Check sheet for the modelled part. Datum: model origin and axes. Units: mm. A direction names the side the tool comes from. Coordinates: 2 decimals unless noted, no trailing zeros. Loops run counter-clockwise (first coordinate to the right, second up) from the corner with the lowest first, then second, coordinate; pieces in that order, holes last. Notation, with made-up numbers: (-6.75, 60.25) - (24.25, 60.25) arc R20 ccw to (24.25, 65.25) - close; hole circle Ø3 at (22.5, -10.75). An arc over 180 degrees is marked (long way). Answer as a JSON object with one key per item and string values. Group by question number.
from build123d import *

# Parameters (mm, degrees)
SKETCH1_R           = 45.72
BOSS_EXTRUDE1_DEPTH = 15.24
SKETCH2_R           = 2.794
CUT_EXTRUDE1_DEPTH  = 67.4296199
CUT_EXTRUDE2_START  = 38.1
SKETCH3_R           = 1.5875
CUT_EXTRUDE2_DEPTH  = 15.24
CIRPATTERN1_COUNT   = 4
SKETCH4_W           = 5.08
SKETCH4_H           = 17.78
SKETCH4_W_2         = 12.7
SKETCH4_H_2         = 5.08
CUT_EXTRUDE3_DEPTH  = 67.429620068


with BuildPart() as part:
    # Sketch1 → Boss-Extrude1 (new body)
    with BuildSketch(Plane.XY):
        with Locations(Location((0, 0, 0), (0, 0, 180))):
            Circle(SKETCH1_R)
    extrude(amount=BOSS_EXTRUDE1_DEPTH)

    # Sketch2 → Cut-Extrude1 (cut, through all)
    with BuildSketch(Plane.XY.offset(15.24)):
        with Locations((-28.575, 0)):
            Circle(SKETCH2_R)
        with Locations((28.575, 0)):
            Circle(SKETCH2_R)
    extrude(amount=-CUT_EXTRUDE1_DEPTH, mode=Mode.SUBTRACT)

    # Sketch3 → Cut-Extrude2 (cut)
    with BuildSketch(Plane(origin=(0, 0, 0), x_dir=(1, 0, 0), z_dir=(0, 1, 0)).offset(CUT_EXTRUDE2_START)):
        with Locations(Location((0, -7.62, 0), (0, 0, 90))):
            Circle(SKETCH3_R)
    cut_extrude2 = extrude(amount=CUT_EXTRUDE2_DEPTH, mode=Mode.SUBTRACT)

    # CirPattern1: Cut-Extrude2 ×4 about axis
    cirpattern1_axis = Axis((0, 0, 0), (0, 0, 1))
    for i in range(1, CIRPATTERN1_COUNT):
        add(cut_extrude2.rotate(cirpattern1_axis, i * 360 / CIRPATTERN1_COUNT), mode=Mode.SUBTRACT)

    # Sketch4 → Cut-Extrude3 (cut, through all)
    with BuildSketch(Plane.XY.offset(15.24)):
        with Locations((3.682680903, 17.78)):
            Rectangle(SKETCH4_W, SKETCH4_H)
        with Locations((3.682680903, -17.78)):
            Rectangle(SKETCH4_W, SKETCH4_H)
        with Locations((-11.557319097, 0)):
            Rectangle(SKETCH4_W_2, SKETCH4_H_2)
    extrude(amount=-CUT_EXTRUDE3_DEPTH, mode=Mode.SUBTRACT)


solid = part.part
1. Gauge pin test, flat ends, axial feed: pin 1 (8 mm diameter, centred on y = 18, z = 11.5, fed in from +X); pin 2 (5.5 mm diameter, centred on x = 4.5, z = 11, fed in from +Y); pin 3 (7.5 mm diameter, centred on y = 18, z = 11, fed in from -X). Record the tip position at first contact, or that the pin passes through.
2. Access from +Z, -Z, +X, -X, +Y, -Y to the whole of each face (thin tool, end or side, straight path). Record for faces 4 (the face through (-38.1, 0, 8)), 5 (the face through (38.1, 0, 8)), 6 (the face through (1.073, -41.857, 8.79)), 7 (the face through (-12, 2.54, 8)), 8 (the face through (1, -1, 15.24)).
3. Sectioned sample at A-A on y = 0. Record the cut outline in (x, z).
4. Sectioned sample at D-D on y = -11.5. Record the cut outline in (x, z).
5. Sectioned sample at C-C on z = 11.5. Record the cut outline in (x, y) (3 decimals), plus the area to 3 significant figures.
6. Sectioned sample at B-B on x = 0. Record the cut outline in (y, z), plus the area to 3 significant figures.
7. Release check for a two-part mould opening along X. For faces 1 (the face through (-41.857, -0.477, 6.106)), 2 (the face through (1.55, 41.86, 7.96)), 3 (the face through (36.28, 27.82, 7.51)) record: released by +X, released by -X, zero draft, split by the parting line, or undercut.
8. Material ranges on line 1 (Z direction, x = 0, y = -40.5); line 2 (X direction, y = -1, z = 7); line 3 (Y direction, x = 3, z = 8.5), recorded low to high.
Answers follow:
{
 "1": {"pin 1": "stops at x = 43.52", "pin 2": "stops at y = 45.69", "pin 3": "stops at x = -43.44"},
 "2": {"face 4": "-X", "face 5": "+X", "face 6": "-Y", "face 7": "+Z, -Z", "face 8": "+Z, +X, -X, +Y, -Y"},
 "3": {"outline": "(-45.72, 0) - (-31.37, 0) - (-31.37, 15.24) - (-45.72, 15.24) - (-45.72, 9.21) - (-38.1, 9.21) - (-38.1, 6.03) - (-45.72, 6.03) - close; (-25.78, 0) - (-17.91, 0) - (-17.91, 15.24) - (-25.78, 15.24) - close; (-5.21, 0) - (25.78, 0) - (25.78, 15.24) - (-5.21, 15.24) - close; (31.37, 0) - (45.72, 0) - (45.72, 6.03) - (38.1, 6.03) - (38.1, 9.21) - (45.72, 9.21) - (45.72, 15.24) - (31.37, 15.24) - close"},
 "4": {"outline": "(-44.25, 0) - (1.14, 0) - (1.14, 15.24) - (-44.25, 15.24) - close; (6.22, 0) - (44.25, 0) - (44.25, 15.24) - (6.22, 15.24) - close"},
 "5": {"outline": "circle Ø91.44 at (0, 0); hole circle Ø5.588 at (-28.575, 0); hole (-17.907, -2.54) - (-5.207, -2.54) - (-5.207, 2.54) - (-17.907, 2.54) - close; hole (1.143, -26.67) - (6.223, -26.67) - (6.223, -8.89) - (1.143, -8.89) - close; hole (1.143, 8.89) - (6.223, 8.89) - (6.223, 26.67) - (1.143, 26.67) - close; hole circle Ø5.588 at (28.575, 0)", "area": "6,270 mm^2"},
 "6": {"outline": "(-45.72, 0) - (45.72, 0) - (45.72, 6.03) - (38.1, 6.03) - (38.1, 9.21) - (45.72, 9.21) - (45.72, 15.24) - (-45.72, 15.24) - (-45.72, 9.21) - (-38.1, 9.21) - (-38.1, 6.03) - (-45.72, 6.03) - close", "area": "1,350 mm^2"},
 "7": {"face 1": "zero draft", "face 2": "undercut", "face 3": "split by the parting line"},
 "8": {"line 1": "z = 0 to 6.03, 9.21 to 15.24", "line 2": "x = -38.1 to -31.18, -25.97 to -17.91, -5.21 to 25.97, 31.18 to 38.1", "line 3": "y = -45.62 to -26.67, -8.89 to 8.89, 26.67 to 45.62"}
}
